Verification items for the finished model (mm, model axes). A direction names the side the tool comes from. Round coordinates to 2 decimals unless told otherwise and drop trailing zeros. Write each loop counter-clockwise with the first axis right and the second up, starting at its lowest first coordinate (ties: lowest second). Pieces come first, ordered by that corner, then holes. Notation, with made-up numbers: M 53,-15.5 L 98,-15.5 A20 ccw 98,5.5 Z; hole C 51,76.25 d3. An arc over 180 degrees is marked long. One line per item, written item: value. Start each with the question number.
Item 1: Draft check along Z on faces 1 (the face through (0.061, 15.027, -45.683)), 2 (the face through (19.06, 15.03, -11.95)), 3 (the face through (-10.812, 15.453, 0.932)). Enter one of: +Z half, -Z half, draft (parallel to the pull), parting line (faces both ways), or undercut.
Item 2: Section check C-C, the plane y = 7. State how many separate pieces and enclosed holes the cut face has, then the cut area to 3 significant figures.
Item 3: Tool access check on faces 4 (the face through (17.457, 15.027, -30.88)), 5 (the face through (35, 15, -9.666)), 6 (the face through (-14.365, 15.453, -33.261)). Record the directions out of +Z, -Z, +X, -X, +Y, -Y that give a thin tool (end or side, any length) a straight path to the whole face; none if there is none.
Item 4: Section check B-B, the plane z = -3.5. Record the cut outline in (x, y), then the cut area to 3 significant figures.
Item 5: Thickness scan on probe 1 along Z at (x, y) = (22, 12); probe 2 along X at (y, z) = (16, -29); probe 3 along Z at (x, y) = (14.5, 24.5). Record the ranges inside material, lowest first. Write a range as from..to.
Item 6: Section check A-A, the plane x = 23.5. Record the cut outline in (y, z), then the cut area to 3 significant figures.
Item 7: Gauge pin test, flat ends, axial feed: pin 1 (6 mm diameter, centred on y = 16.5, z = -15, fed in from +X); pin 2 (3 mm diameter, centred on y = 3.5, z = -43, fed in from +X); pin 3 (5 mm diameter, centred on y = 7.5, z = -36, fed in from +X). Record the tip position at first contact, or that the pin passes through.
from build123d import *

# Parameters (mm, degrees)
SKETCH1_R           = 4.7625
BOSS_EXTRUDE2_DEPTH = 30.48
FILLET1_R           = 2.54


with BuildPart() as part:
    # Sketch1 → Boss-Extrude2 (new body)
    with BuildSketch(Plane(origin=(0, 0, 0), x_dir=(1, 0, 0), z_dir=(0, 1, 0))):
        with BuildLine():
            Line((45.005946436, 2.027668921), (45.515150945, -1.656575462))
            Line((45.515150945, -1.656575462), (-11.575660389, -1.656575462))
            Line((-11.575660389, -1.656575462), (-11.575660389, 25.36121668))
            Line((-11.575660389, 25.36121668), (-14.280396301, 33.422664026))
            ThreePointArc((-14.280396301, 33.422664026), (-17.000257473, 44.802695642), (-5.367910813, 46.064153357))
            Line((-5.367910813, 46.064153357), (5.377854414, 45.31005212))
            Line((5.377854414, 45.31005212), (22.451182043, 35.66511967))
            ThreePointArc((22.451182043, 35.66511967), (18.704388059, 18.178130753), (34.432464589, 9.665736544))
            Line((34.432464589, 9.665736544), (37.367878813, 9.665736544))
            Line((37.367878813, 9.665736544), (45.005946436, 2.027668921))
        make_face()
        with Locations((-11.678835755, 40.598351677)):
            Circle(SKETCH1_R, mode=Mode.SUBTRACT)
        with BuildLine():
            Line((16.202668925, 27.801375987), (18.746230839, 34.046195278))
            ThreePointArc((18.746230839, 34.046195278), (18.80575079, 34.818433424), (18.405670977, 35.481630621))
            ThreePointArc((18.405670977, 35.481630621), (3.288167743, 38.370043483), (-6.637910813, 26.607611872))
            Line((-6.637910813, 26.607611872), (-6.637910813, 1.27))
            ThreePointArc((-6.637910813, 1.27), (-6.265936425, 0.371974388), (-5.367910813, 0))
            Line((-5.367910813, 0), (41.091115974, 0))
            ThreePointArc((41.091115974, 0), (42.264718256, 0.784657148), (41.988123028, 2.169043017))
            Line((41.988123028, 2.169043017), (35.775365429, 8.367731265))
            ThreePointArc((35.775365429, 8.367731265), (35.139277633, 8.711596588), (34.418608086, 8.652550432))
            ThreePointArc((34.418608086, 8.652550432), (18.894618686, 12.123517004), (16.202668925, 27.801375987))
        make_face(mode=Mode.SUBTRACT)
    extrude(amount=BOSS_EXTRUDE2_DEPTH)

    # Fillet1
    fillet1_edges = [part.edges().sort_by_distance(p)[0] for p in [
        (45.515150945, 15.24, 1.656575462),
        (-11.575660389, 15.24, 1.656575462),
        (-11.575660389, 15.24, -25.36121668),
        (-14.280396301, 15.24, -33.422664026),
        (-5.367910813, 15.24, -46.064153357),
        (5.377854414, 15.24, -45.31005212),
        (22.451182043, 15.24, -35.66511967),
        (37.367878813, 15.24, -9.665736544),
    ]]
    fillet(fillet1_edges, radius=FILLET1_R)


solid = part.part
Response values:
1. face 1: -Z half
1. face 2: undercut
1. face 3: +Z half
2. separate pieces: 1
2. enclosed holes: 2
2. area: 639 mm2
3. face 4: +Y, -Y
3. face 5: -Z, +X, +Y, -Y
3. face 6: +Z, -X, +Y, -Y
4. outline: M -11.58,0 L -6.64,0 L -6.64,30.48 L -11.58,30.48 Z; M 40.65,0 L 43.53,0 L 43.53,30.48 L 40.65,30.48 Z
4. area: 238 mm2
5. probe 1: z = -13.59..-9.66, 0..1.66
5. probe 2: x = -12.8..-6.02, 16.69..18.06
5. probe 3: z = -40.16..-37.96, 0..1.66
6. outline: M 0,-12.34 L 30.48,-12.34 L 30.48,-8.89 L 0,-8.89 Z; M 0,0 L 30.48,0 L 30.48,1.66 L 0,1.66 Z
6. area: 156 mm2
7. pin 1: stops at x = 23.99
7. pin 2: stops at x = 12.12
7. pin 3: stops at x = 20.94
